Read the model definition and answer for the solid it produces. Units are mm, in the model's axes. A direction names the side the tool comes from. Coordinates: 2 decimals unless noted, no trailing zeros. Write each loop counter-clockwise with the first axis right and the second up, starting at its lowest first coordinate (ties: lowest second). Pieces come first, ordered by that corner, then holes.
Item 1: Each of these flat-tipped pins is pushed along its axis until it touches: P1, Ø2.5, axis at x = 0, z = 11, coming from the -Y side; P2, Ø2, axis at x = -4, y = 1.5, coming from the +Z side; P3, Ø4.5, axis at x = -11, z = 0, coming from the +Y side; P4, Ø3, axis at x = -10.5, y = -1.5, coming from the +Z side. Where does it stop, or does it pass through?
Item 2: Section A-A (x = 0) is taken. Give the vertices of the cut face in (y, z) (3 decimals), then the cut area to 3 significant figures.
Item 3: Section B-B (z = -11) is taken. Give the vertices of the cut face in (x, y) (3 decimals), then the cut area to 3 significant figures.
Item 4: Straight lines are drawn through the part: probe 1 along Z at (x, y) = (-9, 0.5); probe 2 along Z at (x, y) = (7.25, -1.25); probe 3 along X at (y, z) = (1.5, -1.25). For each, find the intervals that lie inside material, in ascending order.
Item 5: Section D-D (x = -11) is taken. Give the vertices of the cut face in (y, z) (3 decimals).
Item 6: Determine the mould class of faces 1 (the face through (-6, -3.175, -3)), 2 (the face through (-8.092, -0.624, 9.194)) for opening direction X: released by +X, released by -X, zero draft, split by the parting line, or undercut.
Item 7: Section C-C (y = 1.25) is taken. State how many separate pieces and enclosed holes the cut face has, then the cut area to 3 significant figures.
Item 8: A tool of negligible diameter and unlimited length cuts with its end or side. For faces 3 (the face through (-5.525, 0.044, 3.131)), 4 (the face through (-5.1, 3.175, -4.2)), from which of +Z, -Z, +X, -X, +Y, -Y can it reach the whole face along a straight path? Write none if from no direction.
from build123d import *

# Parameters (mm, degrees)
SKETCH1_R                        = 13.97
BOSS_EXTRUDE1_DEPTH              = 3.175
M2_5_CLEARANCE_HOLE1_D           = 2.9
M2_5_CLEARANCE_HOLE1_CSINK_D     = 5.25
M2_5_CLEARANCE_HOLE1_CSINK_ANGLE = 90
CIRPATTERN1_COUNT                = 8


with BuildPart() as part:
    # Sketch1 → Boss-Extrude1 (new, symmetric)
    with BuildSketch(Plane(origin=(0, 0, 0), x_dir=(1, 0, 0), z_dir=(0, 1, 0))):
        with Locations(Location((0, 0, 0), (0, 0, 270))):
            Circle(SKETCH1_R)
        Polygon((3.666174209, 6.35), (-3.666174209, 6.35), (-7.332348419, 0), (-3.666174209, -6.35), (3.666174209, -6.35), (7.332348419, 0), align=None, mode=Mode.SUBTRACT)
    extrude(amount=BOSS_EXTRUDE1_DEPTH, both=True)

    # M2.5 Clearance Hole1 (through all)
    with Locations(Plane(origin=(0, 3.175, 0), x_dir=(1, 0, 0), z_dir=(0, 1, 0))):
        with Locations((0, 11)):
            m2_5_clearance_hole1 = CounterSinkHole(M2_5_CLEARANCE_HOLE1_D / 2, M2_5_CLEARANCE_HOLE1_CSINK_D / 2, counter_sink_angle=M2_5_CLEARANCE_HOLE1_CSINK_ANGLE)

    # CirPattern1: M2.5 Clearance Hole1 ×8 about axis
    cirpattern1_axis = Axis((0, 0, 0), (0, 1, 0))
    for i in range(1, CIRPATTERN1_COUNT):
        add(m2_5_clearance_hole1.rotate(cirpattern1_axis, i * 360 / CIRPATTERN1_COUNT), mode=Mode.SUBTRACT)


solid = part.part
Established:
1. P1: passes through
1. P2: stops at z = 13.64
1. P3: stops at y = 2.8
1. P4: stops at z = 10.68
2. outline: (-3.175, -13.97) - (3.175, -13.97) - (3.175, -13.625) - (2, -12.45) - (-3.175, -12.45) - close; (-3.175, -9.55) - (2, -9.55) - (3.175, -8.375) - (3.175, -6.35) - (-3.175, -6.35) - close; (-3.175, 6.35) - (3.175, 6.35) - (3.175, 8.375) - (2, 9.55) - (-3.175, 9.55) - close; (-3.175, 12.45) - (2, 12.45) - (3.175, 13.625) - (3.175, 13.97) - (-3.175, 13.97) - close
2. area: 57.2 mm2
3. outline: (-8.612, -3.175) - (-1.45, -3.175) - (-1.45, 2) - (-2.625, 3.175) - (-8.612, 3.175) - close; (1.45, -3.175) - (8.612, -3.175) - (8.612, 3.175) - (2.625, 3.175) - (1.45, 2) - close
3. area: 89.6 mm2
4. probe 1: z = -10.68 to -8.56, -7 to 7, 8.56 to 10.68
4. probe 2: z = -11.94 to -9.13, -6.43 to -0.14, 0.14 to 6.43, 9.13 to 11.94
4. probe 3: x = -13.91 to -11.73, -10.27 to -6.61, 6.61 to 10.27, 11.73 to 13.91
5. outline: (-3.175, -8.612) - (3.175, -8.612) - (3.175, -2.625) - (2, -1.45) - (-3.175, -1.45) - close; (-3.175, 1.45) - (2, 1.45) - (3.175, 2.625) - (3.175, 8.612) - (-3.175, 8.612) - close
6. face 1: zero draft
6. face 2: undercut
7. separate pieces: 1
7. enclosed holes: 9
7. area: 421 mm2
8. face 3: +Y, -Y
8. face 4: +Z, -Z, +X, -X, +Y
